```python
from build123d import *

# Parameters (mm, degrees)
SKETCH1_R           = 100
BOSS_EXTRUDE1_DEPTH = 85
CUT_EXTRUDE2_DEPTH  = 85
CUT_EXTRUDE17_DEPTH = 144


with BuildPart() as part:
    # Sketch1 → Boss-Extrude1 (new body)
    with BuildSketch(Plane.XY):
        Circle(SKETCH1_R)
    extrude(amount=BOSS_EXTRUDE1_DEPTH)

    # Sketch2 → Cut-Extrude2 (cut)
    with BuildSketch(Plane.XY.offset(85)):
        with BuildLine():
            Line((0, 45), (-10, 45))
            Line((-10, 45), (-10, 25))
            ThreePointArc((-10, 25), (0, -26.925824036), (10, 25))
            Line((10, 25), (10, 45))
            Line((10, 45), (0, 45))
        make_face()
    extrude(amount=-CUT_EXTRUDE2_DEPTH, mode=Mode.SUBTRACT)

    # Sketch3 → Cut-Extrude17 (cut)
    with BuildSketch(Plane.XY):
        with BuildLine():
            Line((4, 80.412826854), (-4, 80.412826854))
            ThreePointArc((-4, 80.412826854), (-8.212095444, 89.574227067), (-9.987492178, 99.5))
            ThreePointArc((-9.987492178, 99.5), (0, 110), (9.987492178, 99.5))
            ThreePointArc((9.987492178, 99.5), (8.212095444, 89.574227067), (4, 80.412826854))
        make_face()
        with BuildLine():
            Line((28.653156129, 75.241074996), (21.044703998, 77.713210951))
            ThreePointArc((21.044703998, 77.713210951), (19.869791537, 87.727829396), (21.248521423, 97.716428185))
            ThreePointArc((21.248521423, 97.716428185), (33.991869381, 104.616216792), (40.245860457, 91.543818557))
            ThreePointArc((40.245860457, 91.543818557), (35.490125306, 82.652475292), (28.653156129, 75.241074996))
        make_face()
        with BuildLine():
            Line((50.501541697, 62.704202481), (44.029405742, 67.4064845))
            ThreePointArc((44.029405742, 67.4064845), (46.006684882, 77.294020547), (50.4045817, 86.36769155))
            ThreePointArc((50.4045817, 86.36769155), (64.656377752, 88.991869381), (66.564683506, 74.626690331))
            ThreePointArc((66.564683506, 74.626690331), (59.294134429, 67.640123362), (50.501541697, 62.704202481))
        make_face()
        with BuildLine():
            Line((67.4064845, 44.029405742), (62.704202481, 50.501541697))
            ThreePointArc((62.704202481, 50.501541697), (67.640123362, 59.294134429), (74.626690331, 66.564683506))
            ThreePointArc((74.626690331, 66.564683506), (88.991869381, 64.656377752), (86.36769155, 50.4045817))
            ThreePointArc((86.36769155, 50.4045817), (77.294020547, 46.006684882), (67.4064845, 44.029405742))
        make_face()
        with BuildLine():
            Line((77.713210951, 21.044703998), (75.241074996, 28.653156129))
            ThreePointArc((75.241074996, 28.653156129), (82.652475292, 35.490125306), (91.543818557, 40.245860457))
            ThreePointArc((91.543818557, 40.245860457), (104.616216792, 33.991869381), (97.716428185, 21.248521423))
            ThreePointArc((97.716428185, 21.248521423), (87.727829396, 19.869791537), (77.713210951, 21.044703998))
        make_face()
        with BuildLine():
            Line((80.412826854, -4), (80.412826854, 4))
            ThreePointArc((80.412826854, 4), (89.574227067, 8.212095444), (99.5, 9.987492178))
            ThreePointArc((99.5, 9.987492178), (110, 0), (99.5, -9.987492178))
            ThreePointArc((99.5, -9.987492178), (89.574227067, -8.212095444), (80.412826854, -4))
        make_face()
        with BuildLine():
            Line((75.241074996, -28.653156129), (77.713210951, -21.044703998))
            ThreePointArc((77.713210951, -21.044703998), (87.727829396, -19.869791537), (97.716428185, -21.248521423))
            ThreePointArc((97.716428185, -21.248521423), (104.616216792, -33.991869381), (91.543818557, -40.245860457))
            ThreePointArc((91.543818557, -40.245860457), (82.652475292, -35.490125306), (75.241074996, -28.653156129))
        make_face()
        with BuildLine():
            Line((62.704202481, -50.501541697), (67.4064845, -44.029405742))
            ThreePointArc((67.4064845, -44.029405742), (77.294020547, -46.006684882), (86.36769155, -50.4045817))
            ThreePointArc((86.36769155, -50.4045817), (88.991869381, -64.656377752), (74.626690331, -66.564683506))
            ThreePointArc((74.626690331, -66.564683506), (67.640123362, -59.294134429), (62.704202481, -50.501541697))
        make_face()
        with BuildLine():
            Line((44.029405742, -67.4064845), (50.501541697, -62.704202481))
            ThreePointArc((50.501541697, -62.704202481), (59.294134429, -67.640123362), (66.564683506, -74.626690331))
            ThreePointArc((66.564683506, -74.626690331), (64.656377752, -88.991869381), (50.4045817, -86.36769155))
            ThreePointArc((50.4045817, -86.36769155), (46.006684882, -77.294020547), (44.029405742, -67.4064845))
        make_face()
        with BuildLine():
            Line((21.044703998, -77.713210951), (28.653156129, -75.241074996))
            ThreePointArc((28.653156129, -75.241074996), (35.490125306, -82.652475292), (40.245860457, -91.543818557))
            ThreePointArc((40.245860457, -91.543818557), (33.991869381, -104.616216792), (21.248521423, -97.716428185))
            ThreePointArc((21.248521423, -97.716428185), (19.869791537, -87.727829396), (21.044703998, -77.713210951))
        make_face()
        with BuildLine():
            Line((-4, -80.412826854), (4, -80.412826854))
            ThreePointArc((4, -80.412826854), (8.212095444, -89.574227067), (9.987492178, -99.5))
            ThreePointArc((9.987492178, -99.5), (0, -110), (-9.987492178, -99.5))
            ThreePointArc((-9.987492178, -99.5), (-8.212095444, -89.574227067), (-4, -80.412826854))
        make_face()
        with BuildLine():
            Line((-28.653156129, -75.241074996), (-21.044703998, -77.713210951))
            ThreePointArc((-21.044703998, -77.713210951), (-19.869791537, -87.727829396), (-21.248521423, -97.716428185))
            ThreePointArc((-21.248521423, -97.716428185), (-33.991869381, -104.616216792), (-40.245860457, -91.543818557))
            ThreePointArc((-40.245860457, -91.543818557), (-35.490125306, -82.652475292), (-28.653156129, -75.241074996))
        make_face()
        with BuildLine():
            Line((-50.501541697, -62.704202481), (-44.029405742, -67.4064845))
            ThreePointArc((-44.029405742, -67.4064845), (-46.006684882, -77.294020547), (-50.4045817, -86.36769155))
            ThreePointArc((-50.4045817, -86.36769155), (-64.656377752, -88.991869381), (-66.564683506, -74.626690331))
            ThreePointArc((-66.564683506, -74.626690331), (-59.294134429, -67.640123362), (-50.501541697, -62.704202481))
        make_face()
        with BuildLine():
            Line((-67.4064845, -44.029405742), (-62.704202481, -50.501541697))
            ThreePointArc((-62.704202481, -50.501541697), (-67.640123362, -59.294134429), (-74.626690331, -66.564683506))
            ThreePointArc((-74.626690331, -66.564683506), (-88.991869381, -64.656377752), (-86.36769155, -50.4045817))
            ThreePointArc((-86.36769155, -50.4045817), (-77.294020547, -46.006684882), (-67.4064845, -44.029405742))
        make_face()
        with BuildLine():
            Line((-77.713210951, -21.044703998), (-75.241074996, -28.653156129))
            ThreePointArc((-75.241074996, -28.653156129), (-82.652475292, -35.490125306), (-91.543818557, -40.245860457))
            ThreePointArc((-91.543818557, -40.245860457), (-104.616216792, -33.991869381), (-97.716428185, -21.248521423))
            ThreePointArc((-97.716428185, -21.248521423), (-87.727829396, -19.869791537), (-77.713210951, -21.044703998))
        make_face()
        with BuildLine():
            Line((-80.412826854, 4), (-80.412826854, -4))
            ThreePointArc((-80.412826854, -4), (-89.574227067, -8.212095444), (-99.5, -9.987492178))
            ThreePointArc((-99.5, -9.987492178), (-110, 0), (-99.5, 9.987492178))
            ThreePointArc((-99.5, 9.987492178), (-89.574227067, 8.212095444), (-80.412826854, 4))
        make_face()
        with BuildLine():
            Line((-75.241074996, 28.653156129), (-77.713210951, 21.044703998))
            ThreePointArc((-77.713210951, 21.044703998), (-87.727829396, 19.869791537), (-97.716428185, 21.248521423))
            ThreePointArc((-97.716428185, 21.248521423), (-104.616216792, 33.991869381), (-91.543818557, 40.245860457))
            ThreePointArc((-91.543818557, 40.245860457), (-82.652475292, 35.490125306), (-75.241074996, 28.653156129))
        make_face()
        with BuildLine():
            Line((-62.704202481, 50.501541697), (-67.4064845, 44.029405742))
            ThreePointArc((-67.4064845, 44.029405742), (-77.294020547, 46.006684882), (-86.36769155, 50.4045817))
            ThreePointArc((-86.36769155, 50.4045817), (-88.991869381, 64.656377752), (-74.626690331, 66.564683506))
            ThreePointArc((-74.626690331, 66.564683506), (-67.640123362, 59.294134429), (-62.704202481, 50.501541697))
        make_face()
        with BuildLine():
            Line((-44.029405742, 67.4064845), (-50.501541697, 62.704202481))
            ThreePointArc((-50.501541697, 62.704202481), (-59.294134429, 67.640123362), (-66.564683506, 74.626690331))
            ThreePointArc((-66.564683506, 74.626690331), (-64.656377752, 88.991869381), (-50.4045817, 86.36769155))
            ThreePointArc((-50.4045817, 86.36769155), (-46.006684882, 77.294020547), (-44.029405742, 67.4064845))
        make_face()
        with BuildLine():
            Line((-21.044703998, 77.713210951), (-28.653156129, 75.241074996))
            ThreePointArc((-28.653156129, 75.241074996), (-35.490125306, 82.652475292), (-40.245860457, 91.543818557))
            ThreePointArc((-40.245860457, 91.543818557), (-33.991869381, 104.616216792), (-21.248521423, 97.716428185))
            ThreePointArc((-21.248521423, 97.716428185), (-19.869791537, 87.727829396), (-21.044703998, 77.713210951))
        make_face()
    extrude(amount=CUT_EXTRUDE17_DEPTH, mode=Mode.SUBTRACT)


solid = part.part
```
The model under review builds one solid part; all positions refer to its coordinate system, in mm. A direction names the side the tool comes from. Give positions to 0.01 mm unless a question says otherwise; leave off trailing zeros. Write each loop counter-clockwise with the first axis right and the second up, starting at its lowest first coordinate (ties: lowest second). Pieces come first, ordered by that corner, then holes. Notation, with made-up numbers: (-3.75, 11.25) -> (23.25, 11.25) arc R13 ccw to (23.25, 20.25) -> close; hole circle Ø3 at (75.25, 73). An arc over 180 degrees is marked (long way). Answer in a Markdown table with one row per item.
1) Mouldability with a two-part tool opening along X and no side actions: class faces 1 (the cylindrical face through (45.47, 89.064, 41.905)), 2 (the cylindrical face through (-89.137, -45.328, 41.905)), 3 (the cylindrical face through (35.572, 82.768, 41.905)) as +X half, -X half, draft (parallel to the pull), parting line (faces both ways), or undercut.
Worked answers:
| item | result |
|---|---|
| face 1 | +X half |
| face 2 | -X half |
| face 3 | undercut |
2) Clearance check with flat-ended pins moving along their axes: P1, Ø2.5, axis at x = -1, z = 50, coming from the +Y side; P2, Ø1.5, axis at y = -77.5, z = 72, coming from the +X side; P3, Ø12, axis at y = -58.5, z = 56.5, coming from the +X side. State where each tip first meets the part, or that it passes through.
Worked answers:
| item | result |
|---|---|
| P1 | y = 80.41 |
| P2 | x = 46.34 |
| P3 | x = 72.26 |
3) For L1, parallel to Y at x = 0, z = 47; L2, parallel to X at y = 0, z = 53; L3, parallel to Y at x = -50.5, z = 63, list the stretches that pass through material, from the lowest coordinate up. Write a range as [from, to].
Worked answers:
| item | result |
|---|---|
| L1 | [-80.41, -26.93], [45, 80.41] |
| L2 | [-80.41, -26.93], [26.93, 80.41] |
| L3 | [-62.71, 62.71] |
4) Add section A-A on x = 0. State the section outline as (y, z) points, plus the area to 3 significant figures.
Worked answers:
| item | result |
|---|---|
| outline | (-80.41, 0) -> (-26.93, 0) -> (-26.93, 85) -> (-80.41, 85) -> close; (45, 0) -> (80.41, 0) -> (80.41, 85) -> (45, 85) -> close |
| area | 7,560 mm² |
5) Tool access review of faces 4 (the cylindrical face through (89.709, -8.254, 41.905)), 5 (the cylindrical face through (-59.408, -67.725, 41.905)), 6 (the cylindrical face through (8.254, 89.709, 41.905)), 7 (the cylindrical face through (-45.96, -77.16, 41.9)), 8 (the cylindrical face through (-89.709, 8.254, 41.905)): name each direction out of +Z, -Z, +X, -X, +Y, -Y from which nothing blocks a thin tool from reaching the whole face with its end or side.
Worked answers:
| item | result |
|---|---|
| face 4 | +Z, -Z, +X |
| face 5 | +Z, -Z, -Y |
| face 6 | +Z, -Z, +Y |
| face 7 | +Z, -Z |
| face 8 | +Z, -Z, -X |
6) Add section B-B on y = 0. State the section outline as (x, z) points, plus the area to 3 significant figures.
Worked answers:
| item | result |
|---|---|
| outline | (-80.41, 0) -> (-26.93, 0) -> (-26.93, 85) -> (-80.41, 85) -> close; (26.93, 0) -> (80.41, 0) -> (80.41, 85) -> (26.93, 85) -> close |
| area | 9,090 mm² |
